Job drawing, mm, ordinate dimensions from the low corner. One solid piece. A direction names the side the tool comes from. Round coordinates to 2 decimals unless told otherwise and drop trailing zeros. Loops run counter-clockwise (first coordinate to the right, second up) from the corner with the lowest first, then second, coordinate; pieces in that order, holes last.
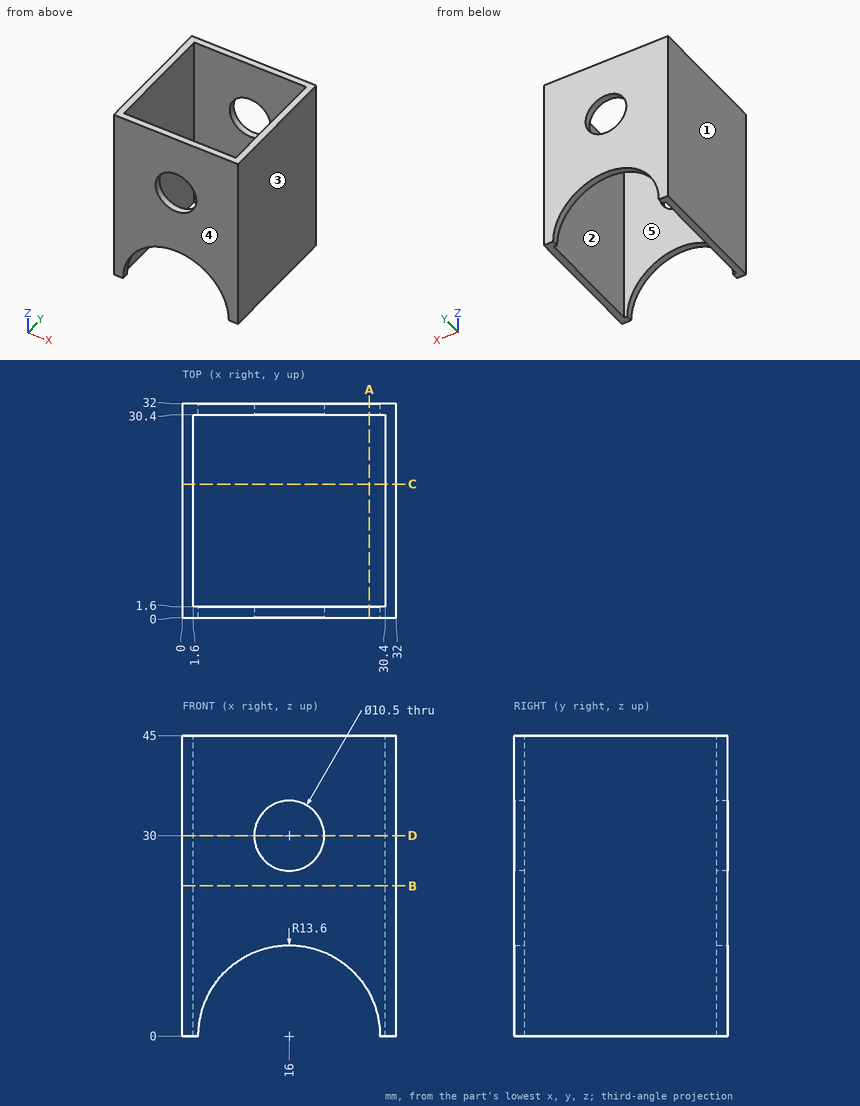
(1) Which spindle directions (+Z, -Z, +X, -X, +Y, -Y) get a long thin tool onto all of the face, cutting with end or side? Do the marked faces 4 and 5. Say none if no direction does.
Responses:
face 4: +Z, -Z, +X, -X, -Y
face 5: +Z, -Z
(2) Slice it at A-A on x = 28. List the corners of the cut face in (y, z), plus the area to 3 significant figures.
Responses:
outline: (0, 6.4) - (1.6, 6.4) - (1.6, 45) - (0, 45) - close; (30.4, 6.4) - (32, 6.4) - (32, 45) - (30.4, 45) - close
area: 124 mm2
(3) Slice it at B-B on z = 22.5. List the corners of the cut face in (x, y).
Responses:
outline: (0, 0) - (32, 0) - (32, 32) - (0, 32) - close; hole (1.6, 1.6) - (30.4, 1.6) - (30.4, 30.4) - (1.6, 30.4) - close
(4) Slice it at C-C on y = 20. List the corners of the cut face in (x, z), plus the area to 3 significant figures.
Responses:
outline: (0, 0) - (1.6, 0) - (1.6, 45) - (0, 45) - close; (30.4, 0) - (32, 0) - (32, 45) - (30.4, 45) - close
area: 144 mm2
(5) Slice it at D-D on z = 30. List the corners of the cut face in (x, y).
Responses:
outline: (0, 0) - (10.75, 0) - (10.75, 1.6) - (1.6, 1.6) - (1.6, 30.4) - (10.75, 30.4) - (10.75, 32) - (0, 32) - close; (21.25, 0) - (32, 0) - (32, 32) - (21.25, 32) - (21.25, 30.4) - (30.4, 30.4) - (30.4, 1.6) - (21.25, 1.6) - close
(6) Pull direction X, two halves, no side cores. Call the marked faces 1, 2 and 3: +X half, -X half, draft (parallel to the pull), parting line (faces both ways), or undercut.
Responses:
face 1: -X half
face 2: undercut
face 3: +X half
(7) Probe line 1 (Y direction, x = 8, z = 20.5); line 2 (X direction, y = 1, z = 30). List the from-to ranges inside material, lowest first.
Responses:
line 1: y = 0 to 1.6, 30.4 to 32
line 2: x = 0 to 10.75, 21.25 to 32
